Part model, mm, in its own coordinate system. A direction names the side the tool comes from. Round coordinates to 2 decimals unless told otherwise and drop trailing zeros. Loops run counter-clockwise (first coordinate to the right, second up) from the corner with the lowest first, then second, coordinate; pieces in that order, holes last.
from build123d import *

# Parameters (mm, degrees)
SKETCH1_W           = 9.525
SKETCH1_H           = 36.5125
BOSS_EXTRUDE1_DEPTH = 1.5
FILLET1_R           = 0.9525
SKETCH2_R           = 1.246
SKETCH2_W           = 6.096
SKETCH2_H           = 2.746
CUT_EXTRUDE1_DEPTH  = 20.104242207


with BuildPart() as part:
    # Sketch1 → Boss-Extrude1 (new, symmetric)
    with BuildSketch(Plane(origin=(0, 0, 0), x_dir=(0, 0, -1), z_dir=(1, 0, 0))):
        Rectangle(SKETCH1_W, SKETCH1_H)
    extrude(amount=BOSS_EXTRUDE1_DEPTH, both=True)

    # Fillet1
    fillet1_edges = [part.edges().sort_by_distance(p)[0] for p in [
        (0, 18.25625, 4.7625),
        (0, 18.25625, -4.7625),
        (0, -18.25625, -4.7625),
        (0, -18.25625, 4.7625),
    ]]
    fillet(fillet1_edges, radius=FILLET1_R)

    # Sketch2 → Cut-Extrude1 (cut, through all)
    with BuildSketch(Plane(origin=(1.5, 0, 0), x_dir=(0, 0, -1), z_dir=(1, 0, 0))):
        with Locations((0, 11.1125)):
            Circle(SKETCH2_R)
        with Locations((0, 15.24)):
            Rectangle(SKETCH2_W, SKETCH2_H)
    cut_extrude1 = extrude(amount=-CUT_EXTRUDE1_DEPTH, mode=Mode.SUBTRACT)

    # Mirror1: Cut-Extrude1 across plane
    add(cut_extrude1.mirror(Plane.ZX), mode=Mode.SUBTRACT)


solid = part.part
1) Drop a flat-ended pin along its axis: pin 1 Ø2 at (y, z) = (11.11, 0) entering from -X. Give the stop position or say it passes through.
Values:
pin 1: passes through
2) Slice it at A-A, the plane z = 0. Give the cut face in (x, y), then the cut area to 3 significant figures.
Values:
outline: (-1.5, -18.26) - (1.5, -18.26) - (1.5, -16.61) - (-1.5, -16.61) - close; (-1.5, -13.87) - (1.5, -13.87) - (1.5, -12.36) - (-1.5, -12.36) - close; (-1.5, -9.87) - (1.5, -9.87) - (1.5, 9.87) - (-1.5, 9.87) - close; (-1.5, 12.36) - (1.5, 12.36) - (1.5, 13.87) - (-1.5, 13.87) - close; (-1.5, 16.61) - (1.5, 16.61) - (1.5, 18.26) - (-1.5, 18.26) - close
area: 78.1 mm2
3) Slice it at C-C, the plane x = -0.75. Give the cut face in (y, z) (1 decimal).
Values:
outline: (-18.3, -3.8) arc R1 ccw to (-17.3, -4.8) - (17.3, -4.8) arc R1 ccw to (18.3, -3.8) - (18.3, 3.8) arc R1 ccw to (17.3, 4.8) - (-17.3, 4.8) arc R1 ccw to (-18.3, 3.8) - close; hole (-16.6, -3) - (-13.9, -3) - (-13.9, 3) - (-16.6, 3) - close; hole circle Ø2.5 at (-11.1, 0); hole circle Ø2.5 at (11.1, 0); hole (13.9, -3) - (16.6, -3) - (16.6, 3) - (13.9, 3) - close
4) Wall check: line 1 along Y through (x, z) = (-0.3, 3); line 2 along Y through (x, z) = (-0.4, 0); line 3 along Z through (x, y) = (-0.7, -14). Give the ranges that are in metal, low to high.
Values:
line 1: y = -18.26 to -16.61, -13.87 to 13.87, 16.61 to 18.26
line 2: y = -18.26 to -16.61, -13.87 to -12.36, -9.87 to 9.87, 12.36 to 13.87, 16.61 to 18.26
line 3: z = -4.76 to -3.05, 3.05 to 4.76
5) Slice it at B-B, the plane y = -10.5. Give the cut face in (x, z).
Values:
outline: (-1.5, -4.76) - (1.5, -4.76) - (1.5, -1.09) - (-1.5, -1.09) - close; (-1.5, 1.09) - (1.5, 1.09) - (1.5, 4.76) - (-1.5, 4.76) - close
6) Mould opens along Y. For faces 1 (the face through (0, 16.613, 0)), 2 (the face through (-0.02, 17.97, 4.49)), 3 (the face through (0, 0, -4.762)) say: released by +Y, released by -Y, zero draft, split by the parting line, or undercut.
Values:
face 1: undercut
face 2: released by +Y
face 3: zero draft
7) Tool access for faces 4 (the face through (0, -18.256, 0)), 5 (the face through (0, -13.867, 0)): list every direction of +Z, -Z, +X, -X, +Y, -Y with a clear straight run to the whole face (end or side of a thin tool).
Values:
face 4: +Z, -Z, +X, -X, -Y
face 5: +X, -X
